Geometry: see drawing. Coordinates: mm, zero at the bounding-box minimum. A direction names the side the tool comes from. Coordinates: 2 decimals unless noted, no trailing zeros. Write each loop counter-clockwise with the first axis right and the second up, starting at its lowest first coordinate (ties: lowest second). Pieces come first, ordered by that corner, then holes. Notation, with made-up numbers: M -3,48.5 L 31,48.5 A33 ccw 31,85.5 Z; hole C 77,83.25 d2. An arc over 180 degrees is marked long. Write item = value, one per line. Start each with the question number.
1. Line query: line 1 along Y through (x, z) = (5, 3.9) (3 decimals); line 2 along Z through (x, y) = (1.25, 5.25); line 3 along X through (y, z) = (7.25, 2.4). Output: solid intervals per line, ascending.
2. Pull-direction query (X, two-part tool) for the marked faces 1, 2 and 3; classes: pulls with the +X half, pulls with the -X half, needs draft (parallel to the pull), parting line crosses it, or undercut.
3. Section query D-D (z = 2.65). Output: boundary loops of the cut face in (x, y) (3 decimals), then the cut area to 3 significant figures.
4. Pin query (flat end, axial travel): pin 1 Ø3.5 at (x, y) = (5, 5) entering from -Z; pin 2 Ø1 at (x, z) = (3.5, 2) entering from +Y; pin 3 Ø1.5 at (y, z) = (8.5, 4) entering from +X. Return the tip coordinate at first contact, or that it passes through.
5. Access query for the marked faces 4 and 5. Directions: +Z, -Z, +X, -X, +Y, -Y. A direction counts if a zero-diameter tool reaches every point of the face in a straight line with its end or side. Return the directions, or none.
6. Section query A-A (y = 5). Output: boundary loops of the cut face in (x, z) (3 decimals).
7. Section query C-C (z = 0.65). Output: boundary loops of the cut face in (x, y).
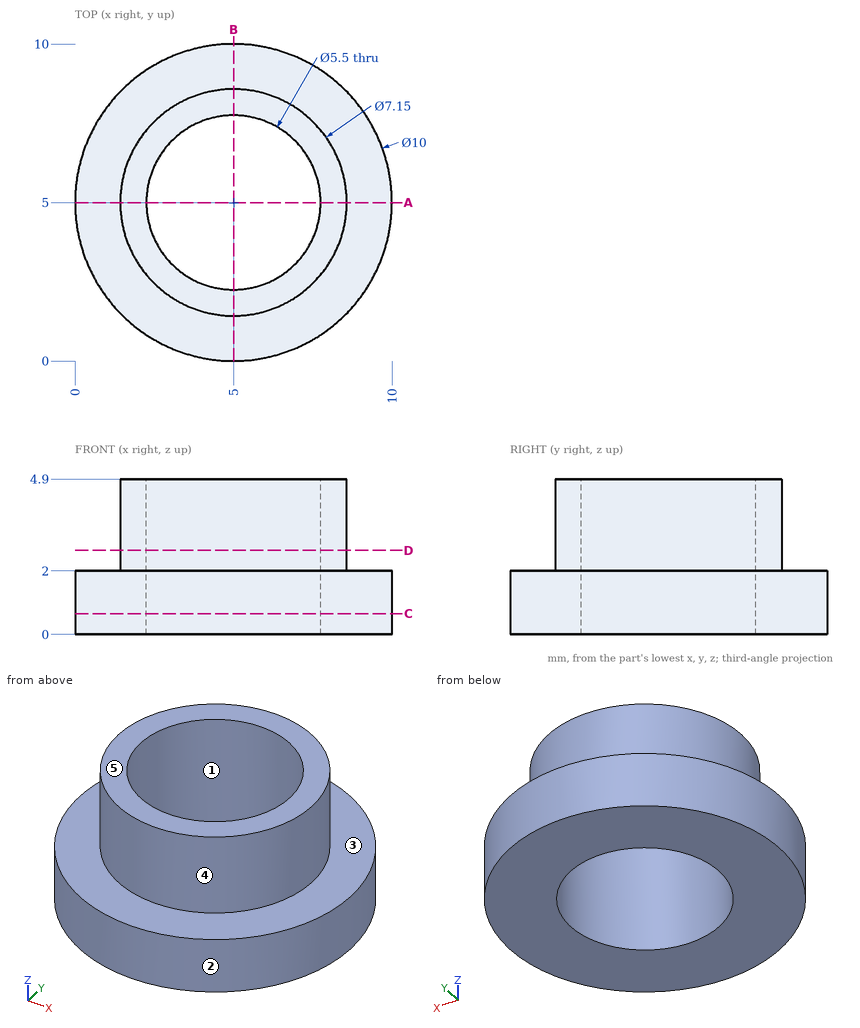
Results are:
q1.line_1 = 1.425 to 2.25, 7.75 to 8.575
q1.line_2 = 0 to 2
q1.line_3 = 2.22 to 3.42, 6.58 to 7.78
q2.face_1 = undercut
q2.face_2 = parting line crosses it
q2.face_3 = needs draft
q3.outline = C 5,5 d7.15; hole C 5,5 d5.5
q3.area = 16.4 mm^2
q4.pin_1 = through
q4.pin_2 = 9.9
q4.pin_3 = 7.28
q5.face_4 = +Z
q5.face_5 = +Z, +X, -X, +Y, -Y
q6.outline = M 0,0 L 2.25,0 L 2.25,4.9 L 1.425,4.9 L 1.425,2 L 0,2 Z; M 7.75,0 L 10,0 L 10,2 L 8.575,2 L 8.575,4.9 L 7.75,4.9 Z
q7.outline = C 5,5 d10; hole C 5,5 d5.5
